Part model, mm, in its own coordinate system. Coordinates: 2 decimals unless noted, no trailing zeros. Write each loop counter-clockwise with the first axis right and the second up, starting at its lowest first coordinate (ties: lowest second). Pieces come first, ordered by that corner, then holes. Notation, with made-up numbers: M 78.5,-14.5 L 114.5,-14.5 A9 ccw 114.5,-0.5 Z; hole C 83.5,36.25 d10. An arc over 180 degrees is marked long. Use a Markdown table: item, result. Add a question column.
Q1. Slice it at B-B on x = -16. Write the cut outline in (y, z).
Q2. Slice it at A-A on z = 3.75. Write the cut outline in (x, y).
Q3. Wall check: L1, parallel to Z at x = -36.5, y = 2.35; L2, parallel to X at y = 1.9, z = -2; L3, parallel to Y at x = 14, z = 3.75. Give the ranges that are in metal, low to high. Write a range as from..to.
Q4. Pin check, flat tips, straight feed: pin 1 Ø2 at (y, z) = (4.5, 2.5) entering from -X; pin 2 Ø5 at (x, z) = (-5.5, 6.5) entering from -Y; pin 3 Ø3 at (x, y) = (76, 4) entering from +Z; pin 4 Ø8 at (x, z) = (-37.5, 2) entering from +Y. Stop position of each tip, or through.
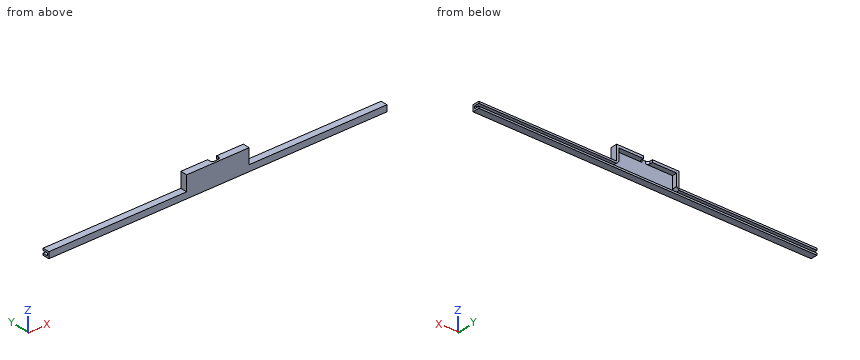
from build123d import *

# Parameters (mm, degrees)
BOSS_EXTRUDE1_DEPTH = 1.5
SKETCH3_W           = 270
SKETCH3_H           = 1.5
BOSS_EXTRUDE2_DEPTH = 4
SKETCH4_W           = 110
SKETCH4_H           = 1.5
BOSS_EXTRUDE3_DEPTH = 4
SKETCH6_W           = 2
SKETCH6_H           = 13.5
BOSS_EXTRUDE5_DEPTH = 4
SKETCH7_W           = 19.5
SKETCH7_H           = 2
BOSS_EXTRUDE6_DEPTH = 4
CHAMFER1_SIZE       = 2
FILLET1_R           = 2


with BuildPart() as part:
    # Sketch1 → Boss-Extrude1 (new body)
    with BuildSketch(Plane(origin=(0, 0, 0), x_dir=(1, 0, 0), z_dir=(0, 1, 0))):
        Polygon((25, 8.5), (135, 8.5), (135, 3.5), (25, 3.5), (25, -8.5), (-25, -8.5), (-25, 3.5), (-135, 3.5), (-135, 8.5), (-25, 8.5), align=None)
    extrude(amount=BOSS_EXTRUDE1_DEPTH)

    # Sketch3 → Boss-Extrude2 (add)
    with BuildSketch(Plane(origin=(0, 1.5, 0), x_dir=(1, 0, 0), z_dir=(0, 1, 0))):
        with Locations((0, 7.75)):
            Rectangle(SKETCH3_W, SKETCH3_H)
    boss_extrude2 = extrude(amount=BOSS_EXTRUDE2_DEPTH)

    # Sketch4 → Boss-Extrude3 (add)
    with BuildSketch(Plane(origin=(0, 1.5, 0), x_dir=(1, 0, 0), z_dir=(0, 1, 0))):
        with Locations((-80, 4.25)):
            Rectangle(SKETCH4_W, SKETCH4_H)
    boss_extrude3 = extrude(amount=BOSS_EXTRUDE3_DEPTH)

    # Mirror1: Boss-Extrude2, Boss-Extrude3 across plane
    add(boss_extrude2.mirror(Plane(origin=(0, 0, 0), x_dir=(0, 0, 1), z_dir=(1, 0, 0))))
    add(boss_extrude3.mirror(Plane(origin=(0, 0, 0), x_dir=(0, 0, 1), z_dir=(1, 0, 0))))

    # Sketch6 → Boss-Extrude5 (add)
    with BuildSketch(Plane(origin=(0, 1.5, 0), x_dir=(1, 0, 0), z_dir=(0, 1, 0))):
        with Locations((-24, -1.75)):
            Rectangle(SKETCH6_W, SKETCH6_H)
        with Locations((24, -1.75)):
            Rectangle(SKETCH6_W, SKETCH6_H)
    extrude(amount=BOSS_EXTRUDE5_DEPTH)

    # Sketch7 → Boss-Extrude6 (add)
    with BuildSketch(Plane(origin=(0, 1.5, 0), x_dir=(1, 0, 0), z_dir=(0, 1, 0))):
        with Locations((-13.25, -7.5)):
            Rectangle(SKETCH7_W, SKETCH7_H)
        with Locations((13.25, -7.5)):
            Rectangle(SKETCH7_W, SKETCH7_H)
    extrude(amount=BOSS_EXTRUDE6_DEPTH)

    # Chamfer1
    chamfer1_edges = [part.edges().sort_by_distance(p)[0] for p in [
        (-23, 3.5, -5),
        (23, 3.5, -5),
    ]]
    chamfer(chamfer1_edges, length=CHAMFER1_SIZE)

    # Fillet1
    fillet1_edges = [part.edges().sort_by_distance(p)[0] for p in [
        (-3.5, 1.5, 7.5),
        (3.5, 1.5, 7.5),
    ]]
    fillet(fillet1_edges, radius=FILLET1_R)


solid = part.part
Recorded:
| question | item | result |
|---|---|---|
| 1 | outline | M 0,-8.5 L 5.5,-8.5 L 5.5,-7 L 1.5,-7 L 1.5,6.5 L 5.5,6.5 L 5.5,8.5 L 0,8.5 Z |
| 2 | outline | M -25,0 L 25,0 L 25,5.5 L 23,5.5 L 23,1.5 L -23,1.5 L -23,5.5 L -25,5.5 Z |
| 3 | L1 | -8.5..-7, -5..-3.5 |
| 3 | L2 | -25..-23, 23..25 |
| 3 | L3 | 0..1.5 |
| 4 | pin 1 | x = -25 |
| 4 | pin 2 | y = 0 |
| 4 | pin 3 | z = -3.5 |
| 4 | pin 4 | through |
